Autodesk Inventor part; units mm, degrees
ref_plane "YZ Plane" through (0, 0, 0) normal (1, 0, 0) x (0, 1, 0)
ref_plane "XZ Plane" through (0, 0, 0) normal (0, 1, 0) x (-1, 0, 0)
ref_plane "XY Plane" through (0, 0, 0) normal (0, 0, 1) x (1, 0, 0)
sketch "Sketch1" plane through (0, 0, 0) normal (0, 1, 0) x (-1, 0, 0)
  line L0 (109.5, 109.5) -> (-109.5, 109.5)
  line L1 (-109.5, 109.5) -> (-109.5, -109.5)
  line L2 (-109.5, -109.5) -> (109.5, -109.5)
  line L3 (109.5, -109.5) -> (109.5, 109.5)
  line L4 (109.5, 109.5) -> (-109.5, -109.5) construction
  line L5 (-109.5, 109.5) -> (109.5, -109.5) construction
  point P0 (0, 0)
  dimension "d0" = 219
extrude "Extrusion1" add sketch "Sketch1" along normal mid plane 3.175
sketch "Sketch2" plane through (0, 1.5875, 0) normal (0, 1, 0) x (1, 0, 0)
  line L0 (-109.5, -109.5) -> (109.5, -109.5) construction
  line L1 (109.5, -109.5) -> (109.5, 109.5) construction
  line L2 (109.5, 109.5) -> (-109.5, 109.5) construction
  line L3 (-109.5, 109.5) -> (-109.5, -109.5) construction
  line L4 (-37.5692, 109.5) -> (-27.5, 97.5)
  line L5 (-27.5, 97.5) -> (27.5, 97.5)
  line L6 (27.5, 97.5) -> (37.5692, 109.5)
  line L7 (37.5692, 109.5) -> (-37.5692, 109.5)
  line L8 (-97.5, -27.5) -> (-97.5, 27.5)
  line L9 (-109.5, -37.5692) -> (-97.5, -27.5)
  line L10 (-109.5, 37.5692) -> (-109.5, -37.5692)
  line L11 (-97.5, 27.5) -> (-109.5, 37.5692)
  line L12 (27.5, -97.5) -> (-27.5, -97.5)
  line L13 (37.5692, -109.5) -> (27.5, -97.5)
  line L14 (-37.5692, -109.5) -> (37.5692, -109.5)
  line L15 (-27.5, -97.5) -> (-37.5692, -109.5)
  line L16 (97.5, 27.5) -> (97.5, -27.5)
  line L17 (109.5, 37.5692) -> (97.5, 27.5)
  line L18 (109.5, -37.5692) -> (109.5, 37.5692)
  line L19 (97.5, -27.5) -> (109.5, -37.5692)
  line L20 (-101.5, 69.5) -> (-101.5, 54.5) construction
  line L21 (-103.5, 69.5) -> (-103.5, 54.5)
  line L22 (-99.5, 54.5) -> (-99.5, 69.5)
  arc A0 (-99.5, 69.5) -> (-103.5, 69.5) centre (-101.5, 69.5) ccw
  arc A1 (-103.5, 54.5) -> (-99.5, 54.5) centre (-101.5, 54.5) ccw
  line L23 (0, 0) -> (-31.1886, 0)
  line L24 (-103.5, -69.5) -> (-103.5, -54.5)
  line L25 (-99.5, -54.5) -> (-99.5, -69.5)
  arc A2 (-103.5, -69.5) -> (-99.5, -69.5) centre (-101.5, -69.5) ccw
  arc A3 (-99.5, -54.5) -> (-103.5, -54.5) centre (-101.5, -54.5) ccw
  point P0 (0, 109.5)
  point P1 (-109.5, 0)
  point P2 (0, -109.5)
  point P3 (109.5, 0)
  point P4 (-101.5, 62)
  dimension "d5" = 55
  dimension "d8" = 360
  dimension "d10" = 195
  dimension "d32" = 4
  dimension "d33" = 15
  dimension "d34" = 52.5
  dimension "d35" = 6
  dimension "d36" = 50
extrude "Extrusion2" cut sketch "Sketch2" against normal blind 3.175
chamfer "Chamfer1" distance 4 angle 45 4 edges at (-109.5, 0, 109.5) (-109.5, 0, -109.5) (109.5, 0, -109.5) (109.5, 0, 109.5)
sketch "Sketch3" plane through (0, 1.5875, 0) normal (0, 1, 0) x (1, 0, 0)
  line L0 (-104.5, -104.5) -> (104.5, -104.5) construction
  line L1 (104.5, -104.5) -> (104.5, 104.5) construction
  line L2 (104.5, 104.5) -> (-104.5, 104.5) construction
  line L3 (-104.5, 104.5) -> (-104.5, -104.5) construction
  line L4 (-104.5, -104.5) -> (104.5, 104.5) construction
  line L5 (104.5, -104.5) -> (-104.5, 104.5) construction
  line L6 (-78.5, 50) -> (-46.5, 50) construction
  line L7 (-78.5, -50) -> (-46.5, -50) construction
  line L8 (46.5, 0) -> (78.5, 0) construction
  point P0 (0, 0)
  point P1 (0, 0)
  dimension "d16" = 209
  dimension "d17" = 209
  dimension "d18" = 32
  dimension "d20" = 46.5
  dimension "d21" = 46.5
  dimension "d22" = 100
  dimension "d23" = 50
  dimension "d24" = 93
hole "Hole1" at (-104.5, 1.5875, -104.5) at (104.5, 1.5875, -104.5) at (104.5, 1.5875, 104.5) at (-104.5, 1.5875, 104.5) direction (0, -1, 0) diameter 3.2 end through all
fillet "Fillet1" radius 1.27 16 edges at (-109.5, 0, -37.5692) (-97.5, 0, -27.5) (-97.5, 0, 27.5) (-109.5, 0, 37.5692) (-27.5, 0, 97.5) (27.5, 0, 97.5) (37.5692, 0, 109.5) (-37.5692, 0, 109.5) (109.5, 0, -37.5692) (97.5, 0, -27.5) (97.5, 0, 27.5) (109.5, 0, 37.5692) (-37.5692, 0, -109.5) (-27.5, 0, -97.5) (27.5, 0, -97.5) (37.5692, 0, -109.5)
sketch "Sketch6" plane through (0, 1.5875, 0) normal (0, 1, 0) x (1, 0, 0)
  point P0 (0, 0)
hole "Hole3" at (0, 1.5875, 0) direction (0, -1, 0) diameter 3 end through all
sketch "Sketch7" plane through (0, -1.5875, 0) normal (0, -1, 0) x (1, 0, 0)
  circle A0 centre (0, 0) radius 1.5
  circle A1 centre (0, 0) radius 1.5
  line L0 (0, 0) -> (-97.5, 0) construction
  line L1 (0, 2) -> (-97.5, 2)
  line L2 (-97.5, -2) -> (0, -2)
  arc A2 (0, -2) -> (0, 2) centre (0, 0) ccw
  arc A3 (-97.5, 2) -> (-97.5, -2) centre (-97.5, 0) ccw
  line L3 (-97.5, 26.9078) -> (-97.5, -26.9078)
  point P0 (-48.75, 0)
  dimension "d59" = 4
extrude "Extrusion4" cut sketch "Sketch7" against normal blind 1.5 contours A2 L2 L3 L1
properties part number "HotBed_Plate_LM6018" material "Aluminum 6061"
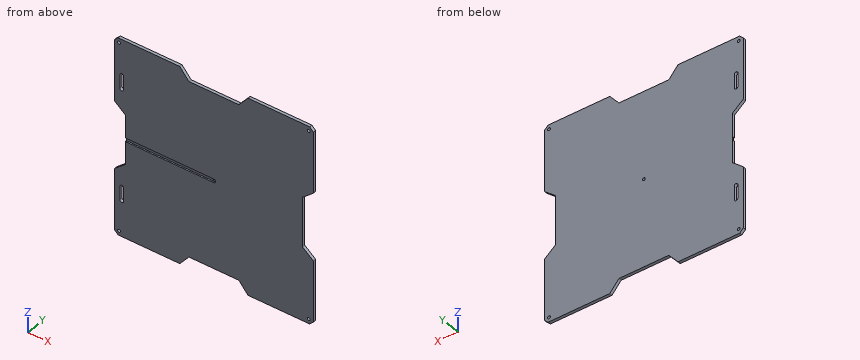
Model file for the job. Use its own axes, mm. Round coordinates to 2 decimals unless told otherwise and drop trailing zeros. Loops run counter-clockwise (first coordinate to the right, second up) from the corner with the lowest first, then second, coordinate; pieces in that order, holes last. Notation, with made-up numbers: (88.25, 31) - (135.25, 31) arc R11 ccw to (135.25, 47) - close; hole circle Ø1 at (-36, 22). An arc over 180 degrees is marked (long way). Write each question's results on one line, items separated by ' | '.
(1) Wall check: L1, parallel to X at y = 1, z = -66; L2, parallel to X at y = 0.7, z = 104.5; L3, parallel to Z at x = -84, y = -1.05. Give the ranges that are in metal, low to high.
Answer below:
L1: x = -109.5 to -103.5, -99.5 to 109.5 | L2: x = -109.5 to -106.1, -102.9 to -33.37, 33.37 to 102.9, 106.1 to 109.5 | L3: z = -109.5 to -2, 2 to 109.5
(2) Saw through at B-B, the plane x = -20.5. List the corners of the cut face in (y, z), then the cut area to 3 significant figures.
Answer below:
outline: (-1.59, -97.5) - (1.59, -97.5) - (1.59, 97.5) - (-1.59, 97.5) - (-1.59, 2) - (-0.09, 2) - (-0.09, -2) - (-1.59, -2) - close | area: 613 mm^2
(3) Pin check, flat tips, straight feed: pin 1 (1.5 mm diameter, centred on x = -20, y = -0.5, fed in from +Z); pin 2 (1.6 mm diameter, centred on y = 0, z = -10.5, fed in from +X); pin 3 (1 mm diameter, centred on y = -0.5, z = 0.5, fed in from -X). Stop position of each tip, or through.
Answer below:
pin 1: stops at z = 97.5 | pin 2: stops at x = 97.5 | pin 3: stops at x = -97.5
(4) Saw through at C-C, the plane y = 0.85. Count the separate pieces of the cut face and the enclosed holes in it, then the cut area to 3 significant figures.
Answer below:
separate pieces: 1 | enclosed holes: 7 | area: 44,600 mm^2
(5) Saw through at A-A, the plane z = -61. List the corners of the cut face in (x, y), then the cut area to 3 significant figures.
Answer below:
outline: (-109.5, -1.59) - (-103.5, -1.59) - (-103.5, 1.59) - (-109.5, 1.59) - close; (-99.5, -1.59) - (109.5, -1.59) - (109.5, 1.59) - (-99.5, 1.59) - close | area: 683 mm^2
